For this review, use the dimensioned drawing (mm, ordinates from the lowest corner) and the shaded views. A direction names the side the tool comes from. Round coordinates to 2 decimals unless told otherwise and drop trailing zeros. Write each loop counter-clockwise with the first axis right and the second up, starting at its lowest first coordinate (ties: lowest second). Pieces come first, ordered by that corner, then holes. Notation, with made-up numbers: (-7, 6) - (48, 6) arc R26 ccw to (48, 45) - close; hole circle Ø7 at (42, -32). An arc over 180 degrees is marked (long way). Return JSON: item names as keys, results as strings.
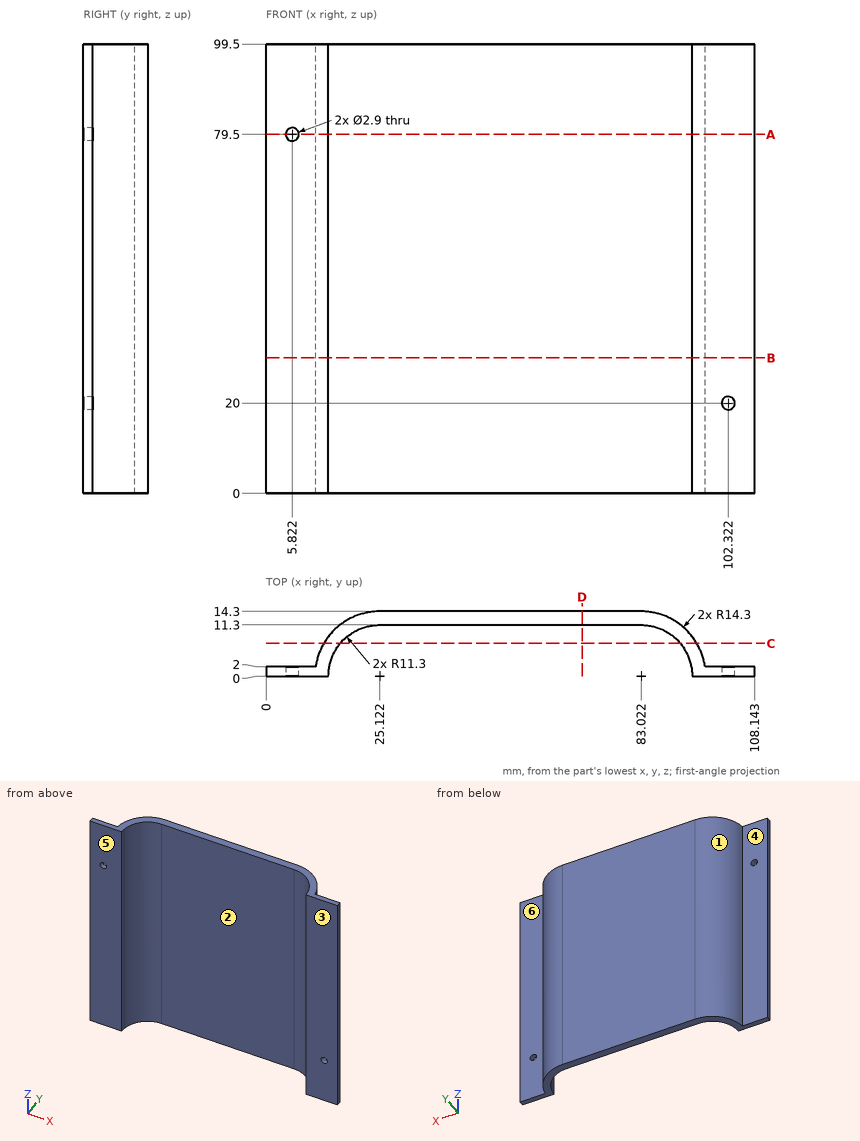
(1) Mouldability with a two-part tool opening along X and no side actions: class the marked faces 1, 2 and 3 as released by +X, released by -X, zero draft, split by the parting line, or undercut.
Filled in:
{"face 1": "released by -X", "face 2": "undercut", "face 3": "zero draft"}
(2) For the marked faces 4, 5 and 6, list the 3-axis set-ups (+Z, -Z, +X, -X, +Y, -Y) from which the entire face can be reached by the end or side of a thin tool; tool diameter is ignored.
Filled in:
{"face 4": "+Z, -Z, -X, +Y", "face 5": "+Z, -Z, +X, -X, -Y", "face 6": "+Z, -Z, +X, +Y"}
(3) Clearance check with flat-ended pins moving along their axes: pin 1 Ø12 at (x, z) = (4.5, 44.5) entering from +Y; pin 2 Ø8 at (x, z) = (75.5, 12) entering from -Y; pin 3 Ø4 at (y, z) = (10.5, 77.5) entering from +X. State where each tip first meets the part, or that it passes through.
Filled in:
{"pin 1": "stops at y = 2", "pin 2": "stops at y = 11.3", "pin 3": "stops at x = 94.52"}
(4) Add section D-D (x = 70). Write out the cut boundary in (y, z).
Filled in:
{"outline": "(11.3, 0) - (14.3, 0) - (14.3, 99.5) - (11.3, 99.5) - close"}
(5) Add section C-C (y = 7.25). Write out the cut boundary in (x, z) (1 decimal), plus the area to 3 significant figures.
Filled in:
{"outline": "(12.8, 0) - (16.5, 0) - (16.5, 99.5) - (12.8, 99.5) - close; (91.7, 0) - (95.3, 0) - (95.3, 99.5) - (91.7, 99.5) - close", "area": "728 mm2"}
(6) Wall thickness on line 1 (X direction, y = 0.75, z = 79.5); line 2 (Y direction, x = 33, z = 94); line 3 (X direction, y = 0.75, z = 32): over which ranges is each line inside the solid? List them lowest first.
Filled in:
{"line 1": "x = 0 to 4.37, 7.27 to 13.85, 94.3 to 108.14", "line 2": "y = 11.3 to 14.3", "line 3": "x = 0 to 13.85, 94.3 to 108.14"}
(7) Add section A-A (z = 79.5). Write out the cut boundary in (x, y), plus the area to 3 significant figures.
Filled in:
{"outline": "(0, 0) - (4.37, 0) - (4.37, 2) - (0, 2) - close; (7.27, 0) - (13.82, 0) arc R11.3 cw to (25.12, 11.3) - (83.02, 11.3) arc R11.3 cw to (94.32, 0) - (108.14, 0) - (108.14, 2) - (97.18, 2) arc R14.3 ccw to (83.02, 14.3) - (25.12, 14.3) arc R14.3 ccw to (10.96, 2) - (7.27, 2) - close", "area": "332 mm2"}
(8) Add section B-B (z = 30). Write out the cut boundary in (x, y).
Filled in:
{"outline": "(0, 0) - (13.82, 0) arc R11.3 cw to (25.12, 11.3) - (83.02, 11.3) arc R11.3 cw to (94.32, 0) - (108.14, 0) - (108.14, 2) - (97.18, 2) arc R14.3 ccw to (83.02, 14.3) - (25.12, 14.3) arc R14.3 ccw to (10.96, 2) - (0, 2) - close"}
